Can you work these out from the model? Positions are in its coordinate system, mm. A direction names the side the tool comes from. Give positions to 0.01 mm unless a question says otherwise; leave off trailing zeros. Order: outer loops, then holes, each group sorted by start corner. A loop starts at its lowest first (then second) coordinate and runs counter-clockwise, first axis right, second up.
Item 1: I want a section at C-C, the plane z = -30. Write out the boundary of the cut face in (x, y), then the cut area to 3 significant figures.
Item 2: If I drill on line 1 along X through (y, z) = (19.25, -28.5) (3 decimals); line 2 along Z through (x, y) = (-27, 6.75); line 3 along X through (y, z) = (4.25, -29.5), over which ranges is the centre line in solid material (lowest first)?
Item 3: If we mould it in two halves opening along Y, with no side actions, what happens to faces 6 (the cylindrical face through (-7.14, 7.9, -40.07)), 7 (the flat face through (-7, 13, -39.291)), 8 (the cylindrical face through (-44.055, 15.402, -30.179))? For each: +Y half, -Y half, draft (parallel to the pull), parting line (faces both ways), or undercut.
Item 4: I want a section at A-A, the plane z = -14. Write out the boundary of the cut face in (x, y) (1 decimal).
Item 5: I want a section at B-B, the plane x = -31. Write out the boundary of the cut face in (y, z), then the cut area to 3 significant figures.
Item 6: I'm going to push flat-ended pins straight in: pin 1 Ø6 at (y, z) = (14, -35) entering from +X; pin 2 Ø8 at (y, z) = (16.5, -23.5) entering from -X (3 decimals); pin 3 Ø0.5 at (x, z) = (-48, -30) entering from +Y; pin 4 Ø3.5 at (x, y) = (-46.04, 5.16) entering from -Z. Where does each tip first touch, or does it pass through?
Item 7: Which directions (+Z, -Z, +X, -X, +Y, -Y) give clear straight access to the entire face, cutting with the end or side of a thin tool? Please do faces 1 (the flat face through (-41.275, 10, -15)), 2 (the flat face through (-41.275, 10, -34)), 3 (the flat face through (0, 10, -34)), 4 (the flat face through (-48.419, 18, -30)), 5 (the flat face through (0, 10, -15)).
```python
from build123d import *

# Parameters (mm, degrees)
BOSS_EXTRUDE1_DEPTH = 20.6375
CUT_EXTRUDE1_DEPTH  = 32.353125
FILLET1_R           = 1
FILLET2_R           = 1
SKETCH3_R           = 4.7625
BOSS_EXTRUDE2_DEPTH = 1.5875
FILLET3_R           = 1
SKETCH4_R           = 3.96875
BOSS_EXTRUDE3_DEPTH = 1.5875


with BuildPart() as part:
    # Sketch1 → Boss-Extrude1 (new body)
    with BuildSketch(Plane(origin=(0, 0, 0), x_dir=(1, 0, 0), z_dir=(0, 1, 0))):
        Polygon((0, 0), (-41.275, 0), (-41.275, 28.971875), (-48.41875, 28.971875), (-48.41875, 31.353125), (-41.275, 31.353125), (-41.275, 37.703125), (0, 37.703125), (0, 31.353125), (7.14375, 31.353125), (7.14375, 28.971875), (0, 28.971875), align=None)
    extrude(amount=BOSS_EXTRUDE1_DEPTH)

    # Sketch2 → Cut-Extrude1 (cut, through all)
    with BuildSketch(Plane(origin=(0, 0, -31.353125), x_dir=(-1, 0, 0), z_dir=(0, 0, -1))):
        with BuildLine():
            Line((-7.14375, 16.271875), (-6.581209729, 16.271875))
            ThreePointArc((-6.581209729, 16.271875), (-2.778125, 15.478125), (-6.581209729, 14.684375))
            Line((-6.581209729, 14.684375), (-7.14375, 14.684375))
            Line((-7.14375, 14.684375), (-7.14375, 16.271875))
        make_face()
        with BuildLine():
            Line((47.856209729, 16.271875), (48.41875, 16.271875))
            Line((48.41875, 16.271875), (48.41875, 14.684375))
            Line((48.41875, 14.684375), (47.856209729, 14.684375))
            ThreePointArc((47.856209729, 14.684375), (44.053125, 15.478125), (47.856209729, 16.271875))
        make_face()
        with BuildLine():
            Line((47.856209729, 4.365625), (48.41875, 4.365625))
            Line((48.41875, 4.365625), (48.41875, 5.953125))
            Line((48.41875, 5.953125), (47.856209729, 5.953125))
            ThreePointArc((47.856209729, 5.953125), (44.053125, 5.159375), (47.856209729, 4.365625))
        make_face()
        with BuildLine():
            Line((-7.14375, 5.953125), (-6.581209729, 5.953125))
            ThreePointArc((-6.581209729, 5.953125), (-2.778125, 5.159375), (-6.581209729, 4.365625))
            Line((-6.581209729, 4.365625), (-7.14375, 4.365625))
            Line((-7.14375, 4.365625), (-7.14375, 5.953125))
        make_face()
    extrude(amount=-CUT_EXTRUDE1_DEPTH, mode=Mode.SUBTRACT)

    # Fillet1
    fillet1_edges = [part.edges().sort_by_distance(p)[0] for p in [
        (7.14375, 20.6375, -30.1625),
        (-48.41875, 0, -30.1625),
        (7.14375, 0, -30.1625),
        (-48.41875, 20.6375, -30.1625),
    ]]
    fillet(fillet1_edges, radius=FILLET1_R)

    # Fillet2
    fillet2_edges = [part.edges().sort_by_distance(p)[0] for p in [
        (-20.6375, 0, 0),
        (-41.275, 0, -14.4859375),
        (-41.275, 0, -34.528125),
        (-20.6375, 0, -37.703125),
        (0, 0, -34.528125),
        (0, 0, -14.4859375),
        (0, 20.6375, -34.528125),
        (-20.6375, 20.6375, -37.703125),
        (0, 10.31875, 0),
        (-41.275, 10.31875, 0),
        (-41.275, 10.31875, -37.703125),
        (0, 10.31875, -37.703125),
        (-41.275, 20.6375, -34.528125),
        (-41.275, 20.6375, -14.4859375),
        (-20.6375, 20.6375, 0),
        (0, 20.6375, -14.4859375),
    ]]
    fillet(fillet2_edges, radius=FILLET2_R)

    # Sketch3 → Boss-Extrude2 (add)
    with BuildSketch(Plane(origin=(0, 0, -37.703125), x_dir=(-1, 0, 0), z_dir=(0, 0, -1))):
        with Locations((10.286875, 10.31875)):
            Circle(SKETCH3_R)
    extrude(amount=BOSS_EXTRUDE2_DEPTH)

    # Fillet3
    fillet3_edges = [part.edges().sort_by_distance(p)[0] for p in [
        (-5.524375, 10.31875, -37.703125),
    ]]
    fillet(fillet3_edges, radius=FILLET3_R)

    # Sketch4 → Boss-Extrude3 (add)
    with BuildSketch(Plane(origin=(0, 0, -39.290625), x_dir=(-1, 0, 0), z_dir=(0, 0, -1))):
        with Locations((10.286875, 10.31875)):
            Circle(SKETCH4_R)
    extrude(amount=BOSS_EXTRUDE3_DEPTH)


solid = part.part
```
Results list:
1. outline: (-48.42, 1) arc R1 ccw to (-47.42, 0) - (6.14, 0) arc R1 ccw to (7.14, 1) - (7.14, 4.37) - (6.58, 4.37) arc R1.98 cw (long way) to (6.58, 5.95) - (7.14, 5.95) - (7.14, 14.68) - (6.58, 14.68) arc R1.98 cw (long way) to (6.58, 16.27) - (7.14, 16.27) - (7.14, 19.64) arc R1 ccw to (6.14, 20.64) - (-47.42, 20.64) arc R1 ccw to (-48.42, 19.64) - (-48.42, 16.27) - (-47.86, 16.27) arc R1.98 cw (long way) to (-47.86, 14.68) - (-48.42, 14.68) - (-48.42, 5.95) - (-47.86, 5.95) arc R1.98 cw (long way) to (-47.86, 4.37) - (-48.42, 4.37) - close
1. area: 1,090 mm2
2. line 1: x = -41.275 to 0
2. line 2: z = -37.7 to 0
2. line 3: x = -48.42 to -47.8, -44.27 to 3, 6.53 to 7.14
3. face 6: parting line
3. face 7: draft
3. face 8: undercut
4. outline: (-41.3, 1) arc R1 ccw to (-40.3, 0) - (-1, 0) arc R1 ccw to (0, 1) - (0, 19.6) arc R1 ccw to (-1, 20.6) - (-40.3, 20.6) arc R1 ccw to (-41.3, 19.6) - close
5. outline: (0, -36.7) arc R1 ccw to (1, -37.7) - (19.64, -37.7) arc R1 ccw to (20.64, -36.7) - (20.64, -1) arc R1 ccw to (19.64, 0) - (1, 0) arc R1 ccw to (0, -1) - close
5. area: 777 mm2
6. pin 1: stops at x = 0
6. pin 2: stops at x = -41.275
6. pin 3: stops at y = 20.58
6. pin 4: passes through
7. face 1: +Z, -X, +Y, -Y
7. face 2: -Z, -X, +Y, -Y
7. face 3: -Z, +X, +Y, -Y
7. face 4: +Z, -Z, -X, +Y, -Y
7. face 5: +Z, +X, +Y, -Y
